from build123d import *

# Parameters (mm, degrees)
SKETCH1_W           = 110
SKETCH1_H           = 114
BOSS_EXTRUDE1_DEPTH = 10
BOSS_EXTRUDE2_DEPTH = 10
SKETCH4_W           = 110
SKETCH4_H           = 7
BOSS_EXTRUDE3_DEPTH = 116.6
SKETCH12_W          = 33
SKETCH12_H          = 7
CUT_EXTRUDE6_DEPTH  = 61.6
SKETCH8_W           = 26
SKETCH8_H           = 30
CUT_EXTRUDE3_DEPTH  = 8
SKETCH9_W           = 13
SKETCH9_H           = 19.5
CUT_EXTRUDE4_DEPTH  = 8
SKETCH10_W          = 17
SKETCH10_H          = 23.5
CUT_EXTRUDE5_DEPTH  = 4
SKETCH6_R           = 3.175
CUT_EXTRUDE1_DEPTH  = 8
BOSS_EXTRUDE5_DEPTH = 10
SKETCH14_R          = 1.75
CUT_EXTRUDE7_DEPTH  = 115
CHAMFER2_SIZE       = 3


with BuildPart() as part:
    # Sketch1 → Boss-Extrude1 (new body)
    with BuildSketch(Plane(origin=(0, 0, 0), x_dir=(1, 0, 0), z_dir=(0, 1, 0))):
        Rectangle(SKETCH1_W, SKETCH1_H)
    extrude(amount=-BOSS_EXTRUDE1_DEPTH)

    # Sketch3 → Boss-Extrude2 (add)
    with BuildSketch(Plane(origin=(0, 0, 0), x_dir=(1, 0, 0), z_dir=(0, 1, 0))):
        Polygon((-55, -50), (-55, -57), (-10, -57), (-10, 57), (-55, 57), (-55, 50), (-22, 50), (-22, -50), align=None)
    extrude(amount=BOSS_EXTRUDE2_DEPTH)

    # Sketch4 → Boss-Extrude3 (add)
    with BuildSketch(Plane(origin=(0, 0, 0), x_dir=(1, 0, 0), z_dir=(0, 1, 0))):
        with Locations((0, 53.5)):
            Rectangle(SKETCH4_W, SKETCH4_H)
    extrude(amount=BOSS_EXTRUDE3_DEPTH)

    # Sketch12 → Cut-Extrude6 (cut)
    with BuildSketch(Plane(origin=(0, 116.6, 0), x_dir=(1, 0, 0), z_dir=(0, 1, 0))):
        with Locations((-38.5, 53.5)):
            Rectangle(SKETCH12_W, SKETCH12_H)
    extrude(amount=-CUT_EXTRUDE6_DEPTH, mode=Mode.SUBTRACT)

    # Sketch8 → Cut-Extrude3 (cut, through all)
    with BuildSketch(Plane.XY.offset(-50)):
        with Locations((11, 15)):
            Rectangle(SKETCH8_W, SKETCH8_H)
    extrude(amount=-CUT_EXTRUDE3_DEPTH, mode=Mode.SUBTRACT)

    # Sketch9 → Cut-Extrude4 (cut, through all)
    with BuildSketch(Plane.XY.offset(-50)):
        with Locations((43.5, 12.75)):
            Rectangle(SKETCH9_W, SKETCH9_H)
    extrude(amount=-CUT_EXTRUDE4_DEPTH, mode=Mode.SUBTRACT)

    # Sketch10 → Cut-Extrude5 (cut)
    with BuildSketch(Plane.XY.offset(-50)):
        with Locations((43.5, 12.75)):
            Rectangle(SKETCH10_W, SKETCH10_H)
    extrude(amount=-CUT_EXTRUDE5_DEPTH, mode=Mode.SUBTRACT)

    # Sketch6 → Cut-Extrude1 (cut, through all)
    with BuildSketch(Plane.XY.offset(-50)):
        with Locations((-5, 101.6)):
            Circle(SKETCH6_R)
        with Locations((40, 101.6)):
            Circle(SKETCH6_R)
        with Locations((-5, 66.6)):
            Circle(SKETCH6_R)
        with Locations((40, 66.6)):
            Circle(SKETCH6_R)
    extrude(amount=-CUT_EXTRUDE1_DEPTH, mode=Mode.SUBTRACT)

    # Sketch11 → Boss-Extrude5 (add)
    with BuildSketch(Plane(origin=(55, 0, 0), x_dir=(0, 0, -1), z_dir=(1, 0, 0))):
        Polygon((57, 116.6), (50, 116.6), (-57, 0), (-57, -10), (57, -10), align=None)
    extrude(amount=BOSS_EXTRUDE5_DEPTH)

    # Sketch14 → Cut-Extrude7 (cut, through all)
    with BuildSketch(Plane(origin=(0, 0, -57), x_dir=(-1, 0, 0), z_dir=(0, 0, -1))):
        with Locations((-29, 15)):
            Circle(SKETCH14_R)
        with Locations((7, 15)):
            Circle(SKETCH14_R)
    extrude(amount=-CUT_EXTRUDE7_DEPTH, mode=Mode.SUBTRACT)

    # Chamfer2
    chamfer2_edges = [part.edges().sort_by_distance(p)[0] for p in [
        (-16, 10, -50),
    ]]
    chamfer(chamfer2_edges, length=CHAMFER2_SIZE)


solid = part.part
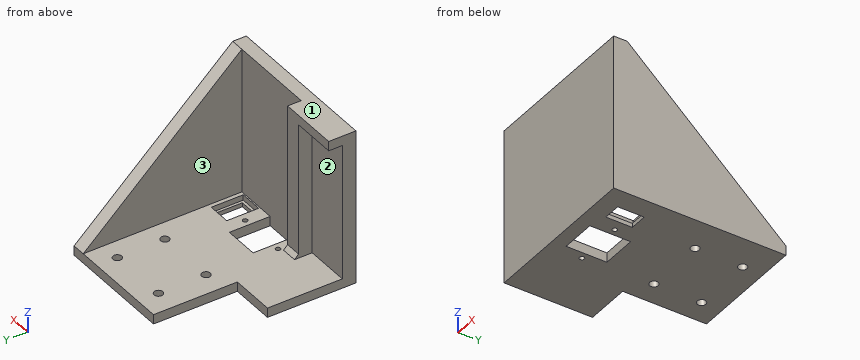
Read the model definition and answer for the solid it produces. Units are mm, in the model's axes. Face numbers are marked on the shaded views. Coordinates: 2 decimals unless noted, no trailing zeros. Loops run counter-clockwise (first coordinate to the right, second up) from the corner with the lowest first, then second, coordinate; pieces in that order, holes last.
Q1. The part is cut by section A-A on x = 29. Write down the section's boundary in (y, z).
Q2. Each of these flat-tipped pins is pushed along its axis until it touches: pin 1 Ø2 at (x, z) = (1, 5.5) entering from +Y; pin 2 Ø10 at (x, y) = (40, 101.6) entering from +Z. Where does it stop, or does it pass through?
Q3. The part is cut by section B-B on y = 101.6. Write down the section's boundary in (x, z) (3 decimals), and give its area (3 significant figures).
Q4. The part is cut by section C-C on x = -45.5. Write down the section's boundary in (y, z).
Q5. The mould has two halves that part along Z. Classify the marked faces 1, 2 and 3: +Z half, -Z half, draft (parallel to the pull), parting line (faces both ways), or undercut.
Q6. The part is cut by section D-D on y = 15. Write down the section's boundary in (x, z) (3 decimals), and give its area (3 significant figures).
Q7. Consider probe 1 along Y at (x, z) = (40, -52.75) (3 decimals); probe 2 along Y at (x, z) = (-5, -53.5) (3 decimals); probe 3 along X at (y, z) = (57.5, -51). Determine where each line is inside the solid, lowest interval first.
Results below:
1. outline: (-10, -57) - (13.25, -57) - (13.25, -50) - (0, -50) - (0, 57) - (-10, 57) - close; (16.75, -57) - (116.6, -57) - (116.6, -50) - (16.75, -50) - close
2. pin 1: stops at y = 0
2. pin 2: stops at z = -50
3. outline: (-22, -57) - (-8.175, -57) - (-8.175, -50) - (-22, -50) - close; (-1.825, -57) - (36.825, -57) - (36.825, -50) - (-1.825, -50) - close; (43.175, -57) - (65, -57) - (65, -36.235) - (55, -36.235) - (55, -50) - (43.175, -50) - close
3. area: 658 mm2
4. outline: (-10, -57) - (55, -57) - (55, -50) - (0, -50) - (0, 50) - (10, 50) - (10, 57) - (-10, 57) - close
5. face 1: +Z half
5. face 2: undercut
5. face 3: draft
6. outline: (-55, -57) - (-8.75, -57) - (-8.75, -50) - (-55, -50) - close; (-5.25, -57) - (-2, -57) - (-2, -50) - (-5.25, -50) - close; (24, -57) - (27.25, -57) - (27.25, -50) - (24, -50) - close; (30.75, -57) - (37, -57) - (37, -54) - (35, -54) - (35, -50) - (30.75, -50) - close; (50, -57) - (65, -57) - (65, 43.235) - (55, 43.235) - (55, -50) - (52, -50) - (52, -54) - (50, -54) - close
6. area: 1,430 mm2
7. probe 1: y = -10 to 1, 24.5 to 63.425, 69.775 to 98.425, 104.775 to 116.6
7. probe 2: y = -10 to 63.425, 69.775 to 98.425, 104.775 to 116.6
7. probe 3: x = -22 to 65
